The listing builds one solid part. Answer for the finished solid, in the listing's coordinates (mm). Coordinates: 2 decimals unless noted, no trailing zeros. Order: outer loops, then holes, each group sorted by start corner. A loop starts at its lowest first (then second) coordinate and runs counter-clockwise, first axis right, second up. Notation, with made-up numbers: (77, 70) -> (97, 70) arc R21 ccw to (97, 83) -> close; hole circle Ø1 at (-29, -11.5). An arc over 180 degrees is marked (long way). Answer in a Markdown table with one row per item. Add a question column.
```python
from build123d import *

# Parameters (mm, degrees)
BOX001027008_W            = 15
BOX001027008_H            = 24
BOX001027008_DEPTH        = 10.6
CYLINDER055_R             = 1.7
CYLINDER055_DEPTH         = 20
CYLINDER055_ROLL_ANGLE    = 90
CYLINDER054_R             = 1.7
CYLINDER054_DEPTH         = 20
CYLINDER054_ROLL_ANGLE    = 90
BOX001021_W               = 16
BOX001021_H               = 4
BOX001021_DEPTH           = 19
CHAMFER002_SIZE           = 4
BOX001023_W               = 14
BOX001023_H               = 9
BOX001023_DEPTH           = 22
BOX001015_W               = 13
BOX001015_H               = 10
BOX001015_DEPTH           = 2
BOX001015_PLACEMENT_ANGLE = 80
BOX001014_W               = 2
BOX001014_H               = 10
BOX001014_DEPTH           = 13
CYLINDER040_R             = 2
CYLINDER040_DEPTH         = 13
CYLINDER040_ROLL_ANGLE    = 90
CYLINDER041_R             = 8
CYLINDER041_DEPTH         = 8
CYLINDER041_ROLL_ANGLE    = 90
COMMON006_PLACEMENT_ANGLE = 25
COMMON005_PITCH_ANGLE     = -20
COMMON004_PITCH_ANGLE     = 10
COMMON007_PITCH_ANGLE     = -35
COMMON003_PITCH_ANGLE     = -5
FUSION061_PLACEMENT_ANGLE = 180
CYLINDER042_R             = 4.6
CYLINDER042_DEPTH         = 10
CYLINDER042_ROLL_ANGLE    = 90
CYLINDER039_R             = 3.2
CYLINDER039_DEPTH         = 10
CYLINDER039_ROLL_ANGLE    = 90
CYLINDER037_R             = 11
CYLINDER037_DEPTH         = 4
CYLINDER037_ROLL_ANGLE    = 90
CYLINDER038_R             = 11
CYLINDER038_DEPTH         = 4
CYLINDER038_ROLL_ANGLE    = 90
BOX001013_W               = 80
BOX001013_H               = 4
BOX001013_DEPTH           = 12
FILLET_R                  = 7
FILLET001_R               = 7
FILLET002_R               = 10
FILLET002_PLACEMENT_ANGLE = 180


with BuildPart() as cube028:
    # Box001027008 → Box001027008 (new body)
    with BuildSketch(Plane(origin=(-11, -13, -38), x_dir=(1, 0, 0), z_dir=(0, 0, 1))):
        with Locations((7.5, 12)):
            Rectangle(BOX001027008_W, BOX001027008_H)
    extrude(amount=BOX001027008_DEPTH)


with BuildPart() as cylinder055:
    # Cylinder055 → Cylinder055 (new body)
    with BuildSketch(Plane.XY):
        Circle(CYLINDER055_R)
    extrude(amount=CYLINDER055_DEPTH)


with BuildPart() as cylinder055_1:
    # Cylinder055 roll: moved
    add(cylinder055.part.rotate(Axis((0, 0, 0), (1, 0, 0)), CYLINDER055_ROLL_ANGLE))


with BuildPart() as cylinder055_2:
    # Cylinder055 placement: moved
    add(cylinder055_1.part.moved(Location((5, 10, -41.5))))


with BuildPart() as fusion075:
    # Cylinder054 → Cylinder054 (new body)
    with BuildSketch(Plane.XY):
        Circle(CYLINDER054_R)
    extrude(amount=CYLINDER054_DEPTH)


with BuildPart() as fusion075_1:
    # Cylinder054 roll: moved
    add(fusion075.part.rotate(Axis((0, 0, 0), (1, 0, 0)), CYLINDER054_ROLL_ANGLE))


with BuildPart() as fusion075_2:
    # Cylinder054 placement: moved
    add(fusion075_1.part.moved(Location((11, 10, -43.5))))

    # Fusion075: union Cylinder055
    add(cylinder055_2.part)


with BuildPart() as cut031:
    # Box001021 → Box001021 (new body)
    with BuildSketch(Plane(origin=(2, -2, -47), x_dir=(1, 0, 0), z_dir=(0, 0, 1))):
        with Locations((8, 2)):
            Rectangle(BOX001021_W, BOX001021_H)
    extrude(amount=BOX001021_DEPTH)

    # Chamfer002
    chamfer002_edges = [cut031.edges().sort_by_distance(p)[0] for p in [
        (18, 0, -47),
    ]]
    chamfer(chamfer002_edges, length=CHAMFER002_SIZE)

    # Cut031: cut Fusion075
    add(fusion075_2.part, mode=Mode.SUBTRACT)


with BuildPart() as cube021:
    # Box001023 → Box001023 (new body)
    with BuildSketch(Plane(origin=(-12, -4, -33), x_dir=(1, 0, 0), z_dir=(0, 0, 1))):
        with Locations((7, 4.5)):
            Rectangle(BOX001023_W, BOX001023_H)
    extrude(amount=BOX001023_DEPTH)


with BuildPart() as cube013:
    # Box001015 → Box001015 (new body)
    with BuildSketch(Plane.XY):
        with Locations((6.5, 5)):
            Rectangle(BOX001015_W, BOX001015_H)
    extrude(amount=BOX001015_DEPTH)


with BuildPart() as cube013_1:
    # Box001015 placement: moved
    add(cube013.part.moved(Location((0, -5, 0))).rotate(Axis((0, -5, 0), (0, -1, 0)), BOX001015_PLACEMENT_ANGLE))


with BuildPart() as common002:
    # Box001014 → Box001014 (new body)
    with BuildSketch(Plane(origin=(0, -5, 0), x_dir=(1, 0, 0), z_dir=(0, 0, 1))):
        with Locations((1, 5)):
            Rectangle(BOX001014_W, BOX001014_H)
    extrude(amount=BOX001014_DEPTH)

    # Common002: intersect Cube013
    add(cube013_1.part, mode=Mode.INTERSECT)


with BuildPart() as cylinder040:
    # Cylinder040 → Cylinder040 (new body)
    with BuildSketch(Plane.XY):
        Circle(CYLINDER040_R)
    extrude(amount=CYLINDER040_DEPTH)


with BuildPart() as cylinder040_1:
    # Cylinder040 roll: moved
    add(cylinder040.part.rotate(Axis((0, 0, 0), (1, 0, 0)), CYLINDER040_ROLL_ANGLE))


with BuildPart() as cylinder040_2:
    # Cylinder040 placement: moved
    add(cylinder040_1.part.moved(Location((0, 7, 0))))


with BuildPart() as cut010:
    # Cylinder041 → Cylinder041 (new body)
    with BuildSketch(Plane.XY):
        Circle(CYLINDER041_R)
    extrude(amount=CYLINDER041_DEPTH)


with BuildPart() as cut010_1:
    # Cylinder041 roll: moved
    add(cut010.part.rotate(Axis((0, 0, 0), (1, 0, 0)), CYLINDER041_ROLL_ANGLE))


with BuildPart() as cut010_2:
    # Cylinder041 placement: moved
    add(cut010_1.part.moved(Location((0, 4, 0))))

    # Cut010: cut Cylinder040
    add(cylinder040_2.part, mode=Mode.SUBTRACT)


with BuildPart() as common006:
    # Common006 base: copy of Cut010
    add(cut010_2.part)

    # Common006: intersect Common002
    add(common002.part, mode=Mode.INTERSECT)


with BuildPart() as common006_1:
    # Common006 placement: moved
    add(common006.part.moved(Location((51.5, 0, 10.598076))).rotate(Axis((51.5, 0, 10.598076), (0, 1, 0)), COMMON006_PLACEMENT_ANGLE))


with BuildPart() as common005:
    # Common005 base: copy of Cut010
    add(cut010_2.part)

    # Common005: intersect Common002
    add(common002.part, mode=Mode.INTERSECT)


with BuildPart() as common005_1:
    # Common005 pitch: moved
    add(common005.part.rotate(Axis((0, 0, 0), (0, 1, 0)), COMMON005_PITCH_ANGLE))


with BuildPart() as common005_2:
    # Common005 placement: moved
    add(common005_1.part.moved(Location((49.223543, 0, 10.897777))))


with BuildPart() as common004:
    # Common004 base: copy of Cut010
    add(cut010_2.part)

    # Common004: intersect Common002
    add(common002.part, mode=Mode.INTERSECT)


with BuildPart() as common004_1:
    # Common004 pitch: moved
    add(common004.part.rotate(Axis((0, 0, 0), (0, 1, 0)), COMMON004_PITCH_ANGLE))


with BuildPart() as common004_2:
    # Common004 placement: moved
    add(common004_1.part.moved(Location((50.776457, 0, 10.897777))))


with BuildPart() as common007:
    # Common007 base: copy of Cut010
    add(cut010_2.part)

    # Common007: intersect Common002
    add(common002.part, mode=Mode.INTERSECT)


with BuildPart() as common007_1:
    # Common007 pitch: moved
    add(common007.part.rotate(Axis((0, 0, 0), (0, 1, 0)), COMMON007_PITCH_ANGLE))


with BuildPart() as common007_2:
    # Common007 placement: moved
    add(common007_1.part.moved(Location((48.5, 0, 10.598076))))


with BuildPart() as common003:
    # Common003 base: copy of Cut010
    add(cut010_2.part)

    # Common003: intersect Common002
    add(common002.part, mode=Mode.INTERSECT)


with BuildPart() as common003_1:
    # Common003 pitch: moved
    add(common003.part.rotate(Axis((0, 0, 0), (0, 1, 0)), COMMON003_PITCH_ANGLE))


with BuildPart() as common003_2:
    # Common003 placement: moved
    add(common003_1.part.moved(Location((50, 0, 11))))


with BuildPart() as strength_slots001:
    # Fusion061 base: copy of Common003
    add(common003_2.part)

    # Fusion061: union Common006, Common005, Common004, Common007
    add(common006_1.part)
    add(common005_2.part)
    add(common004_2.part)
    add(common007_2.part)


with BuildPart() as strength_slots001_1:
    # Fusion061 placement: moved
    add(strength_slots001.part.moved(Location((61, 0, 22))).rotate(Axis((61, 0, 22), (0, 1, 0)), FUSION061_PLACEMENT_ANGLE))


with BuildPart() as cylinder042:
    # Cylinder042 → Cylinder042 (new body)
    with BuildSketch(Plane.XY):
        Circle(CYLINDER042_R)
    extrude(amount=CYLINDER042_DEPTH)


with BuildPart() as cylinder042_1:
    # Cylinder042 roll: moved
    add(cylinder042.part.rotate(Axis((0, 0, 0), (1, 0, 0)), CYLINDER042_ROLL_ANGLE))


with BuildPart() as cylinder042_2:
    # Cylinder042 placement: moved
    add(cylinder042_1.part.moved(Location((11, 5, 15))))


with BuildPart() as strength_slots:
    # Fusion060 base: copy of Common003
    add(common003_2.part)

    # Fusion060: union Common006, Common005, Common004, Common007
    add(common006_1.part)
    add(common005_2.part)
    add(common004_2.part)
    add(common007_2.part)


with BuildPart() as cylinder039:
    # Cylinder039 → Cylinder039 (new body)
    with BuildSketch(Plane.XY):
        Circle(CYLINDER039_R)
    extrude(amount=CYLINDER039_DEPTH)


with BuildPart() as cylinder039_1:
    # Cylinder039 roll: moved
    add(cylinder039.part.rotate(Axis((0, 0, 0), (1, 0, 0)), CYLINDER039_ROLL_ANGLE))


with BuildPart() as cylinder039_2:
    # Cylinder039 placement: moved
    add(cylinder039_1.part.moved(Location((50, 5, 8))))


with BuildPart() as cylinder037:
    # Cylinder037 → Cylinder037 (new body)
    with BuildSketch(Plane.XY):
        Circle(CYLINDER037_R)
    extrude(amount=CYLINDER037_DEPTH)


with BuildPart() as cylinder037_1:
    # Cylinder037 roll: moved
    add(cylinder037.part.rotate(Axis((0, 0, 0), (1, 0, 0)), CYLINDER037_ROLL_ANGLE))


with BuildPart() as cylinder037_2:
    # Cylinder037 placement: moved
    add(cylinder037_1.part.moved(Location((11, 2, 12))))


with BuildPart() as cylinder038:
    # Cylinder038 → Cylinder038 (new body)
    with BuildSketch(Plane.XY):
        Circle(CYLINDER038_R)
    extrude(amount=CYLINDER038_DEPTH)


with BuildPart() as cylinder038_1:
    # Cylinder038 roll: moved
    add(cylinder038.part.rotate(Axis((0, 0, 0), (1, 0, 0)), CYLINDER038_ROLL_ANGLE))


with BuildPart() as cylinder038_2:
    # Cylinder038 placement: moved
    add(cylinder038_1.part.moved(Location((50, 2, 12))))


with BuildPart() as cut_lever_x:
    # Box001013 → Box001013 (new body)
    with BuildSketch(Plane(origin=(0, -2, 0), x_dir=(1, 0, 0), z_dir=(0, 0, 1))):
        with Locations((40, 2)):
            Rectangle(BOX001013_W, BOX001013_H)
    extrude(amount=BOX001013_DEPTH)

    # Fusion059: union Cylinder037, Cylinder038
    add(cylinder037_2.part)
    add(cylinder038_2.part)

    # Fillet
    fillet_edges = [cut_lever_x.edges().sort_by_distance(p)[0] for p in [
        (22, 0, 12),
    ]]
    fillet(fillet_edges, radius=FILLET_R)

    # Fillet001
    fillet001_edges = [cut_lever_x.edges().sort_by_distance(p)[0] for p in [
        (39, 0, 12),
        (61, 0, 12),
    ]]
    fillet(fillet001_edges, radius=FILLET001_R)

    # Cut009: cut Cylinder039
    add(cylinder039_2.part, mode=Mode.SUBTRACT)

    # Cut011: cut strength-slots
    add(strength_slots.part, mode=Mode.SUBTRACT)

    # Cut012: cut Cylinder042
    add(cylinder042_2.part, mode=Mode.SUBTRACT)

    # Cut013: cut strength-slots001
    add(strength_slots001_1.part, mode=Mode.SUBTRACT)

    # Fillet002
    fillet002_edges = [cut_lever_x.edges().sort_by_distance(p)[0] for p in [
        (0, 0, 0),
    ]]
    fillet(fillet002_edges, radius=FILLET002_R)


with BuildPart() as cut_lever_x_1:
    # Fillet002 placement: moved
    add(cut_lever_x.part.moved(Location((75, 0, -16))).rotate(Axis((75, 0, -16), (0, 1, 0)), FILLET002_PLACEMENT_ANGLE))

    # Cut021: cut Cube021
    add(cube021.part, mode=Mode.SUBTRACT)

    # Fusion076: union Cut031
    add(cut031.part)

    # Cut039: cut Cube028
    add(cube028.part, mode=Mode.SUBTRACT)


solid = cut_lever_x_1.part
```
Q1. A cutting plane is placed at C-C (z = -31). State how many separate pieces and enclosed holes the cut face has, then the cut area to 3 significant figures.
Q2. A cutting plane is placed at B-B (z = -24). Determine the outline of the cut face in (x, y).
Q3. Straight lines are drawn through the part: line 1 (Z direction, x = 64, y = -0.05); line 2 (Z direction, x = 11, y = -0.55); line 3 (X direction, y = -1.3, z = -42). For each, find the intervals that lie inside material, in ascending order.
Q4. A cutting plane is placed at A-A (x = 11). Determine the outline of the cut face in (y, z), then the cut area to 3 significant figures.
Q5. Determine the mould class of faces 1 (the face through (20.656, 0.028, -30.659)), 2 (the face through (65.975, 0.028, -38.821)), 3 (the face through (72.15, 0.03, -19.01)) for opening direction Z: +Z half, -Z half, draft (parallel to the pull), parting line (faces both ways), or undercut.
Q6. Given pin 1 (14.5 mm diameter, centred on x = 64, z = -31, fed in from -Y); pin 2 (1.5 mm diameter, centred on y = -1.5, z = -36.5, fed in from +X); pin 3 (1.2 mm diameter, centred on y = -0.5, z = -40.5, fed in from +X); pin 4 (1.2 mm diameter, centred on y = -0.5, z = -33.5, fed in from -X), each flat-ended and moving along its own axis, determine where each tip first touches the part or whether it passes through.
Returned:
| question | item | result |
|---|---|---|
| 1 | separate pieces | 8 |
| 1 | enclosed holes | 0 |
| 1 | area | 159 mm² |
| 2 | outline | (2, -2) -> (21.8, -2) -> (21.8, 2) -> (2, 2) -> close; (28.2, -2) -> (60.12, -2) -> (60.12, 2) -> (28.2, 2) -> close; (60.91, -2) -> (62.09, -2) -> (62.09, 2) -> (60.91, 2) -> close; (62.68, -2) -> (63.74, -2) -> (63.74, 2) -> (62.68, 2) -> close; (64.26, -2) -> (65.32, -2) -> (65.32, 2) -> (64.26, 2) -> close; (65.91, -2) -> (67.09, -2) -> (67.09, 2) -> (65.91, 2) -> close; (67.88, -2) -> (74.8, -2) -> (74.8, 2) -> (67.88, 2) -> close |
| 3 | line 1 | z = -39 to -35.6, -26.4 to -25, -19 to -16 |
| 3 | line 2 | z = -47 to -45.2, -41.8 to -16 |
| 3 | line 3 | x = 2 to 3.38, 6.62 to 10.2, 11.8 to 18 |
| 4 | outline | (-2, -47) -> (2, -47) -> (2, -45.2) -> (-2, -45.2) -> close; (-2, -41.8) -> (2, -41.8) -> (2, -16) -> (-2, -16) -> close |
| 4 | area | 110 mm² |
| 5 | face 1 | undercut |
| 5 | face 2 | -Z half |
| 5 | face 3 | +Z half |
| 6 | pin 1 | stops at y = -2 |
| 6 | pin 2 | stops at x = 71.81 |
| 6 | pin 3 | stops at x = 18 |
| 6 | pin 4 | stops at x = 4 |
